from build123d import *

# Parameters (mm, degrees)
F1_DEPTH = 1.5
F3_DEPTH = 1.2
F4_SIZE  = 0.5
F5_R     = 0.5


with BuildPart() as f1:
    # F0 (on Top) → F1 (new body)
    with BuildSketch(Plane.XY):
        with BuildLine():
            Line((-29.8, -13.5), (29.8, -13.5))
            ThreePointArc((29.8, -13.5), (32.274874, -12.474874), (33.3, -10))
            Line((33.3, -10), (33.3, 10))
            ThreePointArc((33.3, 10), (32.274874, 12.474874), (29.8, 13.5))
            Line((29.8, 13.5), (-29.8, 13.5))
            ThreePointArc((-29.8, 13.5), (-32.274874, 12.474874), (-33.3, 10))
            Line((-33.3, 10), (-33.3, -10))
            ThreePointArc((-33.3, -10), (-32.274874, -12.474874), (-29.8, -13.5))
        make_face()
    extrude(amount=F1_DEPTH)

    # F2 (on face) → F3 (join)
    with BuildSketch(Plane.XY.offset(1.5)):
        Polygon((-15.4, -3), (-15.4, 3), (-21.8, 0), align=None)
        Polygon((21.8, 0), (15.4, 3), (15.4, -3), align=None)
    extrude(amount=F3_DEPTH)

    # F4
    f4_edges = [f1.edges().sort_by_distance(p)[0] for p in [
        (0, -13.5, 0),
        (32.274874, -12.474874, 0),
        (33.3, 0, 0),
        (32.274874, 12.474874, 0),
        (0, 13.5, 0),
        (-32.274874, 12.474874, 0),
        (-33.3, 0, 0),
        (-32.274874, -12.474874, 0),
    ]]
    chamfer(f4_edges, length=F4_SIZE)

    # F5
    f5_edges = [f1.edges().sort_by_distance(p)[0] for p in [
        (-15.4, 0, 2.7),
        (-18.6, 1.5, 2.7),
        (-18.6, -1.5, 2.7),
        (18.6, 1.5, 2.7),
        (15.4, 0, 2.7),
        (18.6, -1.5, 2.7),
        (0, -13.5, 1.5),
        (-32.274874, -12.474874, 1.5),
        (32.274874, -12.474874, 1.5),
        (-33.3, 0, 1.5),
        (33.3, 0, 1.5),
        (-32.274874, 12.474874, 1.5),
        (32.274874, 12.474874, 1.5),
        (0, 13.5, 1.5),
        (-15.4, 0, 1.5),
        (-18.6, 1.5, 1.5),
        (-18.6, -1.5, 1.5),
        (18.6, 1.5, 1.5),
        (15.4, 0, 1.5),
        (18.6, -1.5, 1.5),
    ]]
    fillet(f5_edges, radius=F5_R)


solid = f1.part
CAD build for the part. Positions are in the model's coordinates, mm. Round coordinates to 2 decimals unless told otherwise and drop trailing zeros. Loops run counter-clockwise (first coordinate to the right, second up) from the corner with the lowest first, then second, coordinate; pieces in that order, holes last.
(1) Cut at A-A (y = -8.25). Give the cut face in (x, z).
(2) Drop flat-ended pins along their axis: pin 1 (1.5 mm diameter, centred on y = -5.5, z = 2, fed in from -X); pin 2 (1.5 mm diameter, centred on x = 4.5, y = -6.5, fed in from +Z); pin 3 (1 mm diameter, centred on x = -2.5, z = 1.5, fed in from -Y). Give the stop position or say it passes through.
(3) Cut at B-B (x = -11). Give the cut face in (y, z), plus the area to 3 significant figures.
(4) Wall check: line 1 along Z through (x, y) = (18.5, 11.25); line 2 along X through (y, z) = (-12, 0.45); line 3 along X through (y, z) = (11.5, 0.4). Give the ranges that are in metal, low to high.
(5) Two-plate mould, pull along X, no slides. Class faces 1 (the flat face through (0, 0, 0)), 2 (the flat face through (0, 0, 1.5)), 3 (the cylindrical face through (-32.25, 12.5, 0.75)), 4 (the cylindrical face through (18.495, 1.392, 2.55)): +X half, -X half, draft (parallel to the pull), parting line (faces both ways), or undercut.
Findings below:
1. outline: (-33.3, 0.5) - (-32.8, 0) - (32.8, 0) - (33.3, 0.5) - (33.3, 1) arc R0.5 ccw to (32.8, 1.5) - (-32.8, 1.5) arc R0.5 ccw to (-33.3, 1) - close
2. pin 1: stops at x = -33.23
2. pin 2: stops at z = 1.5
2. pin 3: stops at y = -13.5
3. outline: (-13.5, 0.5) - (-13, 0) - (13, 0) - (13.5, 0.5) - (13.5, 1) arc R0.5 ccw to (13, 1.5) - (-13, 1.5) arc R0.5 ccw to (-13.5, 1) - close
3. area: 40.1 mm2
4. line 1: z = 0 to 1.5
4. line 2: x = -32.61 to 32.61
4. line 3: x = -32.85 to 32.85
5. face 1: draft
5. face 2: undercut
5. face 3: -X half
5. face 4: +X half
